Model file for the job. Use its own axes, mm. A direction names the side the tool comes from. Give positions to 0.01 mm unless a question says otherwise; leave off trailing zeros. Write each loop counter-clockwise with the first axis right and the second up, starting at its lowest first coordinate (ties: lowest second). Pieces come first, ordered by that corner, then holes. Notation, with made-up numbers: (80.25, 53.5) - (136.25, 53.5) arc R28 ccw to (136.25, 85.5) - close; hole circle Ø6 at (-2.5, 32). An arc over 180 degrees is marked (long way). Use a Markdown table: item, result. Add a question column.
```python
from build123d import *

# Parameters (mm, degrees)
SKETCH4_R           = 1.5
SKETCH4_R_2         = 0.5
SKETCH4_R_3         = 2.5
SKETCH4_R_4         = 2
SKETCH4_R_5         = 1
BOSS_EXTRUDE1_DEPTH = 1
SKETCH4_3_R         = 2.5
SKETCH4_3_R_2       = 2
BOSS_EXTRUDE2_DEPTH = 3


with BuildPart() as part:
    # Sketch4 → Boss-Extrude1 (new body)
    # profile 1 of 10: a face of its own
    with BuildSketch(Plane(origin=(0, 0, 0), x_dir=(1, 0, 0), z_dir=(0, 1, 0))):
        with Locations((0, 7)):
            Circle(SKETCH4_R)
        with Locations(Location((0, 7, 0), (0, 0, 270))):
            Circle(SKETCH4_R_2, mode=Mode.SUBTRACT)
    # profile 2 of 10: a face of its own
    with BuildSketch(Plane(origin=(0, 0, 0), x_dir=(1, 0, 0), z_dir=(0, 1, 0))):
        with BuildLine():
            ThreePointArc((-1.5, 2), (0, 2.5), (1.5, 2))
            Line((1.5, 2), (1.5, 7))
            ThreePointArc((1.5, 7), (0, 5.5), (-1.5, 7))
            Line((-1.5, 7), (-1.5, 2))
        make_face()
    # profile 3 of 10: a face of its own
    with BuildSketch(Plane(origin=(0, 0, 0), x_dir=(1, 0, 0), z_dir=(0, 1, 0))):
        with BuildLine():
            ThreePointArc((7, -1.5), (5.5, 0), (7, 1.5))
            Line((7, 1.5), (2, 1.5))
            ThreePointArc((2, 1.5), (2.371708245, 0.790569415), (2.5, 0))
            ThreePointArc((2.5, 0), (2.371708245, -0.790569415), (2, -1.5))
            Line((2, -1.5), (7, -1.5))
        make_face()
    # profile 4 of 10: a face of its own
    with BuildSketch(Plane(origin=(0, 0, 0), x_dir=(1, 0, 0), z_dir=(0, 1, 0))):
        with Locations((7, 0)):
            Circle(SKETCH4_R)
        with Locations(Location((7, 0, 0), (0, 0, 270))):
            Circle(SKETCH4_R_2, mode=Mode.SUBTRACT)
    # profile 5 of 10: a face of its own
    with BuildSketch(Plane(origin=(0, 0, 0), x_dir=(1, 0, 0), z_dir=(0, 1, 0))):
        Circle(SKETCH4_R_3)
        Circle(SKETCH4_R_4, mode=Mode.SUBTRACT)
    # profile 6 of 10: a face of its own
    with BuildSketch(Plane(origin=(0, 0, 0), x_dir=(1, 0, 0), z_dir=(0, 1, 0))):
        Circle(SKETCH4_R_4)
        with Locations(Location((0, 0, 0), (0, 0, 270))):
            Circle(SKETCH4_R_5, mode=Mode.SUBTRACT)
    # profile 7 of 10: a face of its own
    with BuildSketch(Plane(origin=(0, 0, 0), x_dir=(1, 0, 0), z_dir=(0, 1, 0))):
        with Locations((-7, 0)):
            Circle(SKETCH4_R)
        with Locations(Location((-7, 0, 0), (0, 0, 270))):
            Circle(SKETCH4_R_2, mode=Mode.SUBTRACT)
    # profile 8 of 10: a face of its own
    with BuildSketch(Plane(origin=(0, 0, 0), x_dir=(1, 0, 0), z_dir=(0, 1, 0))):
        with BuildLine():
            ThreePointArc((-2, -1.5), (-2.5, 0), (-2, 1.5))
            Line((-2, 1.5), (-7, 1.5))
            ThreePointArc((-7, 1.5), (-5.939339828, 1.060660172), (-5.5, 0))
            ThreePointArc((-5.5, 0), (-5.939339828, -1.060660172), (-7, -1.5))
            Line((-7, -1.5), (-2, -1.5))
        make_face()
    # profile 9 of 10: a face of its own
    with BuildSketch(Plane(origin=(0, 0, 0), x_dir=(1, 0, 0), z_dir=(0, 1, 0))):
        with BuildLine():
            Line((1.5, -7), (1.5, -2))
            ThreePointArc((1.5, -2), (0, -2.5), (-1.5, -2))
            Line((-1.5, -2), (-1.5, -7))
            ThreePointArc((-1.5, -7), (0, -5.5), (1.5, -7))
        make_face()
    # profile 10 of 10: a face of its own
    with BuildSketch(Plane(origin=(0, 0, 0), x_dir=(1, 0, 0), z_dir=(0, 1, 0))):
        with Locations((0, -7)):
            Circle(SKETCH4_R)
        with Locations(Location((0, -7, 0), (0, 0, 270))):
            Circle(SKETCH4_R_2, mode=Mode.SUBTRACT)
    extrude(amount=BOSS_EXTRUDE1_DEPTH)

    # Sketch4_3 → Boss-Extrude2 (add)
    with BuildSketch(Plane(origin=(0, 0, 0), x_dir=(1, 0, 0), z_dir=(0, 1, 0))):
        with Locations(Location((0, 0, 0), (0, 0, 53.130102354))):
            Circle(SKETCH4_3_R)
        with Locations(Location((0, 0, 0), (0, 0, 270))):
            Circle(SKETCH4_3_R_2, mode=Mode.SUBTRACT)
    extrude(amount=BOSS_EXTRUDE2_DEPTH)


solid = part.part
```
(1) Band-saw the part on C-C (y = 0.5). Write the cut outline in (x, z).
(2) Band-saw the part on A-A (x = 0). Write the cut outline in (y, z), then the cut area to 3 significant figures.
(3) Probe probe 1 along X at (y, z) = (0.75, 0); probe 2 along Z at (x, y) = (0, 1.55); probe 3 along X at (y, z) = (0.7, 7). List the from-to ranges inside material, lowest first. Write a range as [from, to].
(4) Band-saw the part on B-B (z = 0). Write the cut outline in (x, y).
(5) Which spindle directions (+Z, -Z, +X, -X, +Y, -Y) get a long thin tool onto all of the face, cutting with end or side? Do faces 4 (the flat face through (-1.5, 0.5, 4.5)), 5 (the flat face through (4.5, 0.5, -1.5)), 6 (the flat face through (4.5, 0.5, 1.5)), 7 (the flat face through (1, 1, 1)), 8 (the flat face through (-1.5, 0.5, -4.5)). Say none if no direction does.
(6) Band-saw the part on D-D (z = 4). Write the cut outline in (x, y), then the cut area to 3 significant figures.
(7) Two-plate mould, pull along Z, no slides. Class faces 1 (the flat face through (-4.5, 0.5, -1.5)), 2 (the cylindrical face through (6.512, 0.493, -0.108)), 3 (the flat face through (1.5, 0.5, 4.5)): +Z half, -Z half, draft (parallel to the pull), parting line (faces both ways), or undercut.
(8) Flat gauge pins, fed straight in: pin 1 (3.5 mm diameter, centred on x = 0.5, z = 5.5, fed in from +Y); pin 2 (5 mm diameter, centred on x = 0, z = 0, fed in from -Y); pin 3 (1.1 mm diameter, centred on y = 0.5, z = -3.5, fed in from +X); pin 4 (1.5 mm diameter, centred on x = 0.5, y = 2.5, fed in from +Z). Where does each tip first touch, or does it go through?
Model answer:
| question | item | result |
|---|---|---|
| 1 | outline | (-7, -1.5) - (-2, -1.5) arc R2.5 ccw to (-1.5, -2) - (-1.5, -7) arc R1.5 ccw to (1.5, -7) - (1.5, -2) arc R2.5 ccw to (2, -1.5) - (7, -1.5) arc R1.5 ccw to (7, 1.5) - (2, 1.5) arc R2.5 ccw to (1.5, 2) - (1.5, 7) arc R1.5 ccw to (-1.5, 7) - (-1.5, 2) arc R2.5 ccw to (-2, 1.5) - (-7, 1.5) arc R1.5 ccw to start; hole circle Ø1 at (-7, 0); hole circle Ø2 at (0, 0); hole circle Ø1 at (0, -7); hole circle Ø1 at (0, 7); hole circle Ø1 at (7, 0) |
| 2 | outline | (0, -8.5) - (1, -8.5) - (1, -7.5) - (0, -7.5) - close; (0, -6.5) - (1, -6.5) - (1, -2.5) - (3, -2.5) - (3, -2) - (1, -2) - (1, -1) - (0, -1) - close; (0, 1) - (1, 1) - (1, 2) - (3, 2) - (3, 2.5) - (1, 2.5) - (1, 6.5) - (0, 6.5) - close; (0, 7.5) - (1, 7.5) - (1, 8.5) - (0, 8.5) - close |
| 2 | area | 15.0 mm^2 |
| 3 | probe 1 | x = [-8.5, -7.5], [-6.5, -1], [1, 6.5], [7.5, 8.5] |
| 3 | probe 2 | z = [-2.5, -2], [2, 2.5] |
| 3 | probe 3 | x = [-1.5, -0.5], [0.5, 1.5] |
| 4 | outline | (-8.5, 0) - (-7.5, 0) - (-7.5, 1) - (-8.5, 1) - close; (-6.5, 0) - (-1, 0) - (-1, 1) - (-2, 1) - (-2, 3) - (-2.5, 3) - (-2.5, 1) - (-6.5, 1) - close; (1, 0) - (6.5, 0) - (6.5, 1) - (2.5, 1) - (2.5, 3) - (2, 3) - (2, 1) - (1, 1) - close; (7.5, 0) - (8.5, 0) - (8.5, 1) - (7.5, 1) - close |
| 5 | face 4 | +Z, -X, +Y, -Y |
| 5 | face 5 | -Z, +X, +Y, -Y |
| 5 | face 6 | +Z, +X, +Y, -Y |
| 5 | face 7 | +Y |
| 5 | face 8 | -Z, -X, +Y, -Y |
| 6 | outline | (-1.5, 0) - (1.5, 0) - (1.5, 1) - (-1.5, 1) - close |
| 6 | area | 3.00 mm^2 |
| 7 | face 1 | -Z half |
| 7 | face 2 | undercut |
| 7 | face 3 | draft |
| 8 | pin 1 | stops at y = 1 |
| 8 | pin 2 | stops at y = 0 |
| 8 | pin 3 | stops at x = 1.5 |
| 8 | pin 4 | stops at z = 2.5 |
